Verification items for the finished model (mm, model axes). Give positions to 0.01 mm unless a question says otherwise; leave off trailing zeros. Loops run counter-clockwise (first coordinate to the right, second up) from the corner with the lowest first, then second, coordinate; pieces in that order, holes last. Notation, with made-up numbers: M 79.5,31 L 91.5,31 A16 cw 91.5,49 Z; hole C 73,-18 d1. An arc over 180 degrees is marked long. Answer in a Markdown table with one row per item.
```python
from build123d import *

# Parameters (mm, degrees)
F1_DEPTH = 10
F2_R     = 4
F3_R     = 5
F4_R     = 5


with BuildPart() as f1:
    # F0 (on Front) → F1 (new body)
    with BuildSketch(Plane.XZ):
        Polygon((4.83675, 1.025512), (0.519318, 4.916923), (-4.515794, 2.013314), (-3.310232, -3.672627), (2.469957, -4.283122), align=None)
    extrude(amount=F1_DEPTH)

    # F2
    f2_edges = [f1.edges().sort_by_distance(p)[0] for p in [
        (-0.420137, -10, -3.977874),
    ]]
    fillet(f2_edges, radius=F2_R)

    # F3
    f3_edges = [f1.edges().sort_by_distance(p)[0] for p in [
        (4.83675, -5, 1.025512),
    ]]
    fillet(f3_edges, radius=F3_R)

    # F4
    f4_edges = [f1.edges().sort_by_distance(p)[0] for p in [
        (-4.515794, -5, 2.013314),
    ]]
    fillet(f4_edges, radius=F4_R)


solid = f1.part
```
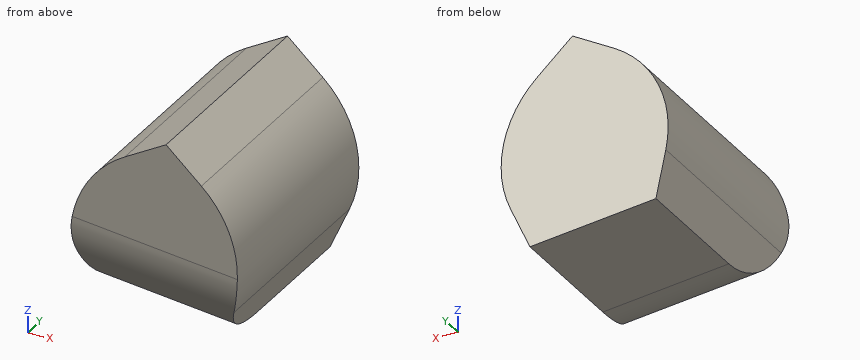
Item 1: Sectioned sample at C-C (y = -6.25). Record the cut outline in (x, z).
Reported:
| item | result |
|---|---|
| outline | M -3.76,-1.54 L -3.31,-3.66 L 2.47,-4.28 L 3.36,-2.29 A5 ccw 2.14,3.46 L 0.52,4.92 L -1.37,3.83 A5 ccw Z |
Item 2: Sectioned sample at D-D (z = 2.75). Record the cut outline in (x, y), and give its area (3 significant figures).
Reported:
| item | result |
|---|---|
| outline | M -2.67,-10 L 2.79,-10 L 2.79,0 L -2.67,0 Z |
| area | 54.5 mm^2 |
Item 3: Go/stop test with flat-tipped pins: pin 1 (3 mm diameter, centred on x = -2.5, y = -4.5, fed in from +Z); pin 2 (2 mm diameter, centred on y = -3.5, z = -0.5, fed in from +X); pin 3 (2 mm diameter, centred on y = -7.5, z = 3.5, fed in from +X). Record where each tip stops, or that it passes through.
Reported:
| item | result |
|---|---|
| pin 1 | stops at z = 4.04 |
| pin 2 | stops at x = 3.79 |
| pin 3 | stops at x = 2.96 |
Item 4: Sectioned sample at A-A (y = -4). Record the cut outline in (x, z), and give its area (3 significant figures).
Reported:
| item | result |
|---|---|
| outline | M -3.76,-1.54 L -3.31,-3.67 L 2.47,-4.28 L 3.36,-2.29 A5 ccw 2.14,3.46 L 0.52,4.92 L -1.37,3.83 A5 ccw Z |
| area | 53.2 mm^2 |
Item 5: Sectioned sample at B-B (z = 4). Record the cut outline in (x, y).
Reported:
| item | result |
|---|---|
| outline | M -1.07,-10 L 1.54,-10 L 1.54,0 L -1.07,0 Z |
Item 6: Scan lines: L1, parallel to X at y = -7.5, z = -0.5; L2, parallel to X at y = -3, z = 1.5; L3, parallel to Z at x = -1.5, y = -7.75. Record each from-to range of solid material in increasing order. Write a range as [from, to].
Reported:
| item | result |
|---|---|
| L1 | x = [-3.87, 3.78] |
| L2 | x = [-3.45, 3.47] |
| L3 | z = [-3.46, 3.75] |
